Design review of the part built by this model. Coordinates are the model's own, in mm. A direction names the side the tool comes from. Round coordinates to 2 decimals unless told otherwise and drop trailing zeros. Order: outer loops, then holes, each group sorted by start corner. A loop starts at its lowest first (then second) coordinate and runs counter-clockwise, first axis right, second up. Notation, with made-up numbers: M 3,-4.5 L 13,-4.5 A23 ccw 13,33.5 Z; hole C 59.25,-24.75 d11. An arc over 180 degrees is marked long. Use a Markdown table: item, result. Add a question column.
(1) Take a section at A-A (z = 32). Write out the cut boundary in (x, y).
(2) The part is to be moulded in two halves that separate along X. For faces 1 (the face through (0, -2.5, 17)), 2 (the face through (1.5, 0.07, -2.96)), 3 (the face through (0.27, -1.22, 31.2)), say which applies: released by +X, released by -X, zero draft, split by the parting line, or undercut.
(3) Machinability: for faces 4 (the face through (-2.175, -1.233, 17.255)), 5 (the face through (1.24, 1.15, 0)), which of the approach directions +Z, -Z, +X, -X, +Y, -Y give a long, thin tool a straight path to every point of the face, cutting with its end or side? Answer none if there is none.
(4) To check wall thickness, follow probe 1 along Y at (x, z) = (0, 31.5); probe 2 along Z at (x, y) = (-2.15, 0.4); probe 3 along Y at (x, z) = (2.5, 24.5). State the ranges of each line that lie inside material, in increasing order. Write a range as from..to.
(5) Take a section at C-C (x = 2.4). Write out the cut boundary in (y, z).
(6) Take a section at B-B (z = 0.5). Write out the cut boundary in (x, y), then the cut area to 3 significant figures.
(7) Take a section at D-D (y = 2). Write out the cut boundary in (x, z), then the cut area to 3 significant figures.
```python
from build123d import *

# Parameters (mm, degrees)
EXTRUDE_1_DEPTH = 35
SKETCH_4_R      = 1.5
EXTRUDE_2_DEPTH = 6
M3X0_5_1_D      = 2.5
M3X0_5_1_DEPTH  = 7.5
M3X0_5_1_TIP    = 0.751075774


with BuildPart() as part:
    # 草圖1 → 填料-伸長1 (new body)
    with BuildSketch(Plane.XY):
        Polygon((-1.443375673, 2.5), (-2.886751346, 0), (-1.443375673, -2.5), (1.443375673, -2.5), (2.886751346, 0), (1.443375673, 2.5), align=None)
    extrude(amount=EXTRUDE_1_DEPTH)

    # 草圖4 → 填料-伸長2 (add)
    with BuildSketch(Plane(origin=(0, 0, 0), x_dir=(-1, 0, 0), z_dir=(0, 0, -1))):
        Circle(SKETCH_4_R)
    extrude(amount=EXTRUDE_2_DEPTH)

    # M3x0.5 螺紋孔1
    with Locations(Plane.XY.offset(35)):
        with Locations((0, 0)):
            Hole(M3X0_5_1_D / 2, depth=M3X0_5_1_DEPTH)
            with Locations((0, 0, -(M3X0_5_1_DEPTH + M3X0_5_1_TIP / 2))):  # 118° drill point
                Cone(0, M3X0_5_1_D / 2, M3X0_5_1_TIP, mode=Mode.SUBTRACT)


solid = part.part
```
Verdict:
| question | item | result |
|---|---|---|
| 1 | outline | M -2.89,0 L -1.44,-2.5 L 1.44,-2.5 L 2.89,0 L 1.44,2.5 L -1.44,2.5 Z; hole C 0,0 d2.5 |
| 2 | face 1 | zero draft |
| 2 | face 2 | split by the parting line |
| 2 | face 3 | undercut |
| 3 | face 4 | +Z, -Z, -X, -Y |
| 3 | face 5 | -Z |
| 4 | probe 1 | y = -2.5..-1.25, 1.25..2.5 |
| 4 | probe 2 | z = 0..35 |
| 4 | probe 3 | y = -0.67..0.67 |
| 5 | outline | M -0.84,0 L 0.84,0 L 0.84,35 L -0.84,35 Z |
| 6 | outline | M -2.89,0 L -1.44,-2.5 L 1.44,-2.5 L 2.89,0 L 1.44,2.5 L -1.44,2.5 Z |
| 6 | area | 21.7 mm^2 |
| 7 | outline | M -1.73,0 L 1.73,0 L 1.73,35 L -1.73,35 Z |
| 7 | area | 121 mm^2 |
